CAD build for the part. Positions are in the model's coordinates, mm. Face numbers are marked on the shaded views. A direction names the side the tool comes from. Round coordinates to 2 decimals unless told otherwise and drop trailing zeros. Order: outer loops, then holes, each group sorted by start corner. A loop starts at its lowest first (then second) coordinate and runs counter-clockwise, first axis right, second up. Notation, with made-up numbers: M 70,17.5 L 105,17.5 A12 ccw 105,31.5 Z; hole C 46.25,33.25 d3. An arc over 180 degrees is marked long. Put each result on its own line as item: value.
```python
from build123d import *

# Parameters (mm, degrees)
ESQUISSE1_R             = 55
ESQUISSE1_R_2           = 48
ESQUISSE1_R_3           = 2.1
BOSS_EXTRU_1_DEPTH      = 64
ENL_V_MAT_EXTRU_1_DEPTH = 101.727354775
CONG_1_R                = 9


with BuildPart() as part:
    # Esquisse1 → Boss.-Extru.1 (new body)
    with BuildSketch(Plane.XY):
        Circle(ESQUISSE1_R)
        Circle(ESQUISSE1_R_2, mode=Mode.SUBTRACT)
        with Locations((0, 51.5)):
            Circle(ESQUISSE1_R_3, mode=Mode.SUBTRACT)
        with Locations((30.270940493, 41.66437521)):
            Circle(ESQUISSE1_R_3, mode=Mode.SUBTRACT)
        with Locations((48.979410589, 15.91437521)):
            Circle(ESQUISSE1_R_3, mode=Mode.SUBTRACT)
        with Locations((48.979410589, -15.91437521)):
            Circle(ESQUISSE1_R_3, mode=Mode.SUBTRACT)
        with Locations((30.270940493, -41.66437521)):
            Circle(ESQUISSE1_R_3, mode=Mode.SUBTRACT)
        with Locations((0, -51.5)):
            Circle(ESQUISSE1_R_3, mode=Mode.SUBTRACT)
        with Locations((-30.270940493, -41.66437521)):
            Circle(ESQUISSE1_R_3, mode=Mode.SUBTRACT)
        with Locations((-48.979410589, -15.91437521)):
            Circle(ESQUISSE1_R_3, mode=Mode.SUBTRACT)
        with Locations((-48.979410589, 15.91437521)):
            Circle(ESQUISSE1_R_3, mode=Mode.SUBTRACT)
        with Locations((-30.270940493, 41.66437521)):
            Circle(ESQUISSE1_R_3, mode=Mode.SUBTRACT)
    extrude(amount=BOSS_EXTRU_1_DEPTH)

    # Esquisse3 → Enlèv. mat.-Extru.1 (cut, through all)
    with BuildSketch(Plane.XY.offset(64)):
        Polygon((0, 0), (60, 43.59255168), (60, -43.59255168), align=None)
    extrude(amount=-ENL_V_MAT_EXTRU_1_DEPTH, mode=Mode.SUBTRACT)

    # Congé1
    # the kernel refuses this fillet: 9 mm, written as the material it takes off along each edge
    with BuildSketch(Plane(origin=(38.83281573, -28.21369211, 82.806493839), x_dir=(0.809016994374856, -0.5877852522925988, 0), z_dir=(0, 0, -1))) as cong_1_piece_1:
        with BuildLine():
            CenterArc((8.3, 8.905616206), CONG_1_R, 188.98865434, 72.706236132)
            Line((-0.589473684, 7.499466278), (-0.767263158, 7.47134328))
            ThreePointArc((-0.767263158, 7.47134328), (-0.327041859, 3.747193897), (-0.18, 0))
            Line((-0.18, 0), (0, -0.18))
            ThreePointArc((0, -0.18), (3.5, -0.18), (6.974, -0.178112324))
            Line((6.974, -0.178112324), (7, 0))
        make_face()
    extrude(amount=101.612987679, mode=Mode.SUBTRACT)
    with BuildSketch(Plane(origin=(38.83281573, 28.21369211, 82.806493839), x_dir=(0.8090169943748586, 0.5877852522925953, 0), z_dir=(0, 0, -1))) as cong_1_piece_2:
        with BuildLine():
            CenterArc((8.3, -8.905616206), CONG_1_R, 98.305109528, 72.706236132)
            Line((-0.589473684, -7.499466278), (-0.767263158, -7.47134328))
            ThreePointArc((-0.767263158, -7.47134328), (-0.327041859, -3.747193897), (-0.18, 0))
            Line((-0.18, 0), (0, 0.18))
            ThreePointArc((0, 0.18), (3.5, 0.18), (6.974, 0.178112324))
            Line((6.974, 0.178112324), (7, 0))
        make_face()
    extrude(amount=101.612987679, mode=Mode.SUBTRACT)


solid = part.part
```
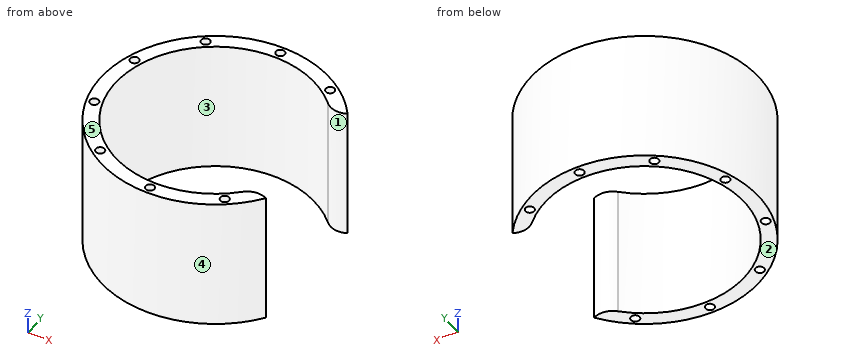
Item 1: Tool access for the marked faces 1 and 2: list every direction of +Z, -Z, +X, -X, +Y, -Y with a clear straight run to the whole face (end or side of a thin tool).
Answers below:
face 1: +Z, -Z
face 2: -Z, +X, -X, +Y, -Y
Item 2: Band-saw the part on B-B on y = -45.5. Give the cut face in (x, z).
Answers below:
outline: M -30.9,0 L -15.29,0 L -15.29,64 L -30.9,64 Z; M 15.29,0 L 30.9,0 L 30.9,64 L 15.29,64 Z
Item 3: Band-saw the part on A-A on x = 18. Give the cut face in (y, z), and give its area (3 significant figures).
Answers below:
outline: M -51.97,0 L -44.5,0 L -44.5,64 L -51.97,64 Z; M 44.5,0 L 51.97,0 L 51.97,64 L 44.5,64 Z
area: 957 mm²
Item 4: Mould opens along Y. For the marked faces 3, 4 and 5 say: pulls with the +Y half, pulls with the -Y half, needs draft (parallel to the pull), parting line crosses it, or undercut.
Answers below:
face 3: undercut
face 4: parting line crosses it
face 5: needs draft
Item 5: Pin check, flat tips, straight feed: P1, Ø12, axis at x = -44.5, z = 21.5, coming from the +Y side; P2, Ø6, axis at y = -21.5, z = 12.5, coming from the +X side; P3, Ø1.5, axis at x = 32.5, z = 23, coming from the -Y side; P4, Ø2.5, axis at x = 0, y = 51.5, coming from the -Z side. Stop position of each tip, or through.
Answers below:
P1: y = 39.28
P2: x = -41.28
P3: y = -44.91
P4: through
Item 6: Band-saw the part on C-C on z = 18.5. State how many separate pieces and enclosed holes the cut face has, and give its area (3 significant figures).
Answers below:
separate pieces: 1
enclosed holes: 8
area: 1,680 mm²
Item 7: Band-saw the part on D-D on x = -0.5. Give the cut face in (y, z).
Answers below:
outline: M -55,0 L -53.54,0 L -53.54,64 L -55,64 Z; M -49.46,0 L -48,0 L -48,64 L -49.46,64 Z; M 48,0 L 49.46,0 L 49.46,64 L 48,64 Z; M 53.54,0 L 55,0 L 55,64 L 53.54,64 Z
Item 8: Probe line 1 along Y through (x, z) = (0, 23); line 2 along Y through (x, z) = (29.5, 22); line 3 along X through (y, z) = (42.5, 36). List the from-to ranges inside material, lowest first. Write a range as [from, to].
Answers below:
line 1: [-55, -53.6], [-49.4, -48], [48, 49.4], [53.6, 55]
line 2: [-46.42, -43.62], [-39.71, -37.86], [37.86, 39.71], [43.62, 46.42]
line 3: [-34.91, -32.2], [-28.34, -22.31], [22.31, 28.34], [32.2, 34.91]
